Verification items for the finished model (mm, model axes). A direction names the side the tool comes from. Round coordinates to 2 decimals unless told otherwise and drop trailing zeros. Loops run counter-clockwise (first coordinate to the right, second up) from the corner with the lowest first, then second, coordinate; pieces in that order, holes last. Notation, with made-up numbers: M 11.5,-24.5 L 32.5,-24.5 A20 ccw 32.5,14.5 Z; hole C -32,81.25 d9. An arc over 180 degrees is marked long. Write item = value, one per line. Start each with the question number.
from build123d import *

# Parameters (mm, degrees)
SKETCH1_W           = 34
SKETCH1_H           = 30
BOSS_EXTRUDE1_DEPTH = 15
SKETCH2_R           = 2.1
CUT_EXTRUDE1_DEPTH  = 6
CHAMFER1_SIZE       = 1


with BuildPart() as part:
    # Sketch1 → Boss-Extrude1 (new body)
    with BuildSketch(Plane.XY):
        Rectangle(SKETCH1_W, SKETCH1_H)
    extrude(amount=BOSS_EXTRUDE1_DEPTH)

    # Sketch2 → Cut-Extrude1 (cut)
    with BuildSketch(Plane(origin=(0, 0, 0), x_dir=(-1, 0, 0), z_dir=(0, 0, -1))):
        with Locations((12, -9)):
            Circle(SKETCH2_R)
        with Locations((12, 9)):
            Circle(SKETCH2_R)
        with Locations((-12, 9)):
            Circle(SKETCH2_R)
        with Locations((-12, -9)):
            Circle(SKETCH2_R)
    extrude(amount=-CUT_EXTRUDE1_DEPTH, mode=Mode.SUBTRACT)

    # Chamfer1
    chamfer1_edges = [part.edges().sort_by_distance(p)[0] for p in [
        (14.1, -9, 0),
        (14.1, 9, 0),
        (-9.9, 9, 0),
        (-9.9, -9, 0),
    ]]
    chamfer(chamfer1_edges, length=CHAMFER1_SIZE)


solid = part.part
1. Section check A-A, the plane y = -9. Enter the section's corners in (x, z), and give its area (3 significant figures).
2. Thickness scan on line 1 (Y direction, x = 12, z = 2); line 2 (X direction, y = 8.5, z = 5.25); line 3 (Z direction, x = -14, y = 9.25). Record the ranges inside material, lowest first.
3. Mould release check, pull along Y, two halves, no side actions. Record for faces 3 (the flat face through (0, -15, 7)), 4 (the cylindrical face through (12.273, 11.082, 3.465)), 5 (the flat face through (0, 0, 15)), 6 (the flat face through (0, 15, 7)): pulls with the +Y half, pulls with the -Y half, needs draft (parallel to the pull), parting line crosses it, or undercut.
4. Gauge pin test, flat ends, axial feed: P1, Ø3.5, axis at x = 12, y = 9, coming from the -Z side; P2, Ø4.5, axis at x = -11.5, y = -9, coming from the -Z side; P3, Ø3.5, axis at x = -12.5, y = 9.5, coming from the -Z side. Record the tip position at first contact, or that the pin passes through.
5. Section check C-C, the plane x = -12. Enter the section's corners in (y, z), and give its area (3 significant figures).
6. Tool access check on faces 1 (the flat face through (17, 0, 7)), 2 (the flat face through (12, 9, 6)). Record the directions out of +Z, -Z, +X, -X, +Y, -Y that give a thin tool (end or side, any length) a straight path to the whole face; none if there is none.
7. Section check B-B, the plane z = 4.75. Enter the section's corners in (x, y), and give its area (3 significant figures).
Computed values:
q1.outline = M -17,0 L -15.1,0 L -14.1,1 L -14.1,6 L -9.9,6 L -9.9,1 L -8.9,0 L 8.9,0 L 9.9,1 L 9.9,6 L 14.1,6 L 14.1,1 L 15.1,0 L 17,0 L 17,15 L -17,15 Z
q1.area = 458 mm2
q2.line_1 = -15 to -11.1, -6.9 to 6.9, 11.1 to 15
q2.line_2 = -17 to -14.04, -9.96 to 9.96, 14.04 to 17
q2.line_3 = 6 to 15
q3.face_3 = pulls with the -Y half
q3.face_4 = undercut
q3.face_5 = needs draft
q3.face_6 = pulls with the +Y half
q4.P1 = 6
q4.P2 = 0.35
q4.P3 = 0.64
q5.outline = M -15,0 L -12.1,0 L -11.1,1 L -11.1,6 L -6.9,6 L -6.9,1 L -5.9,0 L 5.9,0 L 6.9,1 L 6.9,6 L 11.1,6 L 11.1,1 L 12.1,0 L 15,0 L 15,15 L -15,15 Z
q5.area = 398 mm2
q6.face_1 = +Z, -Z, +X, +Y, -Y
q6.face_2 = -Z
q7.outline = M -17,-15 L 17,-15 L 17,15 L -17,15 Z; hole C -12,-9 d4.2; hole C -12,9 d4.2; hole C 12,-9 d4.2; hole C 12,9 d4.2
q7.area = 965 mm2
